Drawing for the job (mm, zero at the part's lowest x, y, z). A direction names the side the tool comes from. Round coordinates to 2 decimals unless told otherwise and drop trailing zeros. Loops run counter-clockwise (first coordinate to the right, second up) from the corner with the lowest first, then second, coordinate; pieces in that order, holes last. Notation, with made-up numbers: M 57,-4.5 L 67,-4.5 A14 cw 67,21.5 Z; hole C 28,0.5 d1. An arc over 180 degrees is marked long. Use a Markdown table: item, result. Add a question column.
Q1. Cut at D-D (y = 16.5). Give the cut face in (x, z) (1 decimal).
Q2. Tool access for the marked faces 4 and 5: list every direction of +Z, -Z, +X, -X, +Y, -Y with a clear straight run to the whole face (end or side of a thin tool).
Q3. Mould opens along Y. For the marked faces 1, 2 and 3 say: +Y half, -Y half, draft (parallel to the pull), parting line (faces both ways), or undercut.
Q4. Cut at A-A (y = 11.75). Give the cut face in (x, z).
Q5. Pin check, flat tips, straight feed: pin 1 (2 mm diameter, centred on x = 8.5, z = 5.5, fed in from -Y); pin 2 (5 mm diameter, centred on x = 29, z = 10, fed in from -Y); pin 3 (4 mm diameter, centred on x = 4.5, z = 3, fed in from -Y) (1 decimal). Stop position of each tip, or through.
Q6. Probe line 1 (X direction, y = 9.5, z = 3) (1 decimal); line 2 (Z direction, x = 25.5, y = 8); line 3 (X direction, y = 12, z = 8.5) (1 decimal). List the from-to ranges inside material, lowest first. Write a range as from..to.
Q7. Cut at B-B (x = 20.5). Give the cut face in (y, z).
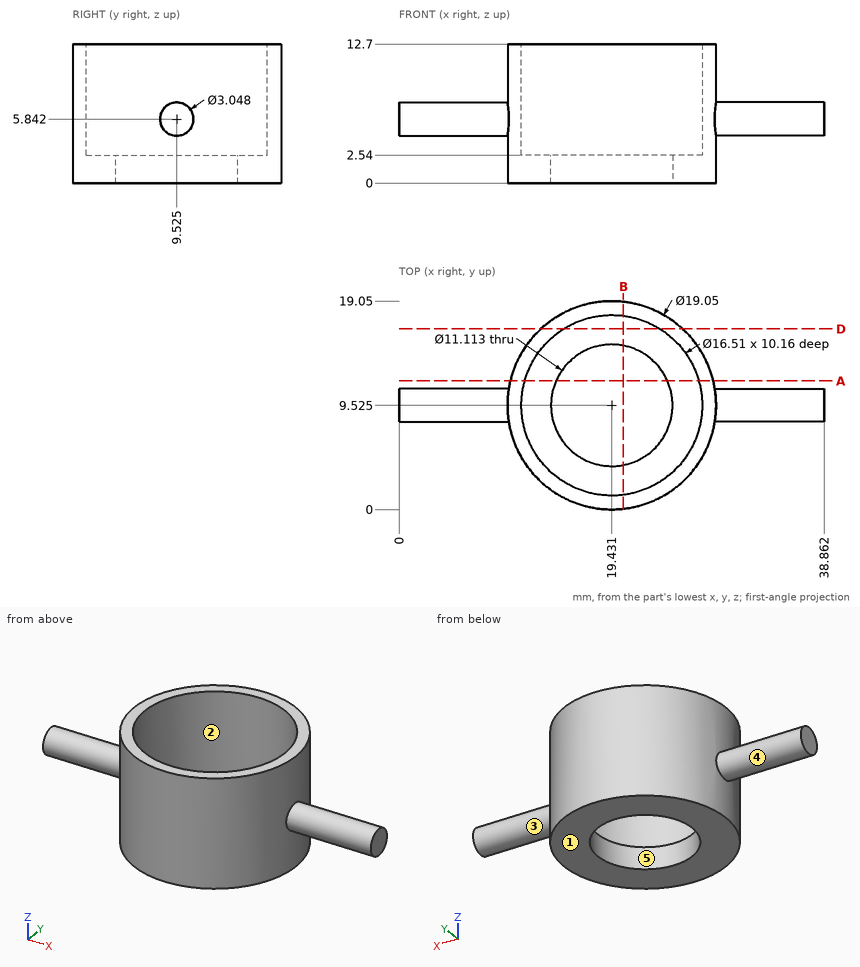
Checked values:
| question | item | result |
|---|---|---|
| 1 | outline | M 12.9,0 L 25.9,0 L 25.9,12.7 L 23.8,12.7 L 23.8,2.5 L 15,2.5 L 15,12.7 L 12.9,12.7 Z |
| 2 | face 4 | -X |
| 2 | face 5 | +Z, -Z |
| 3 | face 1 | draft |
| 3 | face 2 | undercut |
| 3 | face 3 | parting line |
| 4 | outline | M 10.17,0 L 14.34,0 L 14.34,2.54 L 11.48,2.54 L 11.48,12.7 L 10.17,12.7 Z; M 24.52,0 L 28.69,0 L 28.69,12.7 L 27.38,12.7 L 27.38,2.54 L 24.52,2.54 Z |
| 5 | pin 1 | stops at y = 8 |
| 5 | pin 2 | stops at y = 3.14 |
| 5 | pin 3 | stops at y = 8.3 |
| 6 | line 1 | x = 9.9..11.2, 27.7..29 |
| 6 | line 2 | z = 0..2.54 |
| 6 | line 3 | x = 10.2..11.6, 27.3..28.6 |
| 7 | outline | M 0.06,0 L 4.07,0 L 4.07,2.54 L 1.34,2.54 L 1.34,12.7 L 0.06,12.7 Z; M 14.98,0 L 18.99,0 L 18.99,12.7 L 17.71,12.7 L 17.71,2.54 L 14.98,2.54 Z |
